```python
from build123d import *

# Parameters (mm, degrees)
F0_R            = 150
F1_DEPTH        = 15
F3_DEPTH        = 15.001
F3_COPIES_COUNT = 6
F5_DEPTH        = 3
F5_COPIES_COUNT = 6
F6_R            = 25
F6_R_2          = 11.35
F7_DEPTH        = 3
F8_DEPTH        = 15.001


# Not quite as in the source:
# - an extrude ends at something that could not be found from the text; its depth is read off the source's solid
# - a pattern or mirror of a feature is missing from the dataset's text; its kind, count and spacing are read off the source's solid


with BuildPart() as f1:
    # F0 (on Top) → F1 (new body)
    with BuildSketch(Plane.XY):
        Circle(F0_R)
    extrude(amount=F1_DEPTH)

    # F2 (on face) → F3 (cut, through all)
    with BuildSketch(Plane.XY.offset(15)):
        with BuildLine():
            ThreePointArc((0, 120), (-5.3033008589, 117.8033008589), (-7.5, 112.5))
            Line((-7.5, 112.5), (-7.5, 27.5))
            ThreePointArc((-7.5, 27.5), (-5.3033008589, 22.1966991411), (0, 20))
            Line((0, 20), (0, 120))
        make_face()
        with BuildLine():
            ThreePointArc((7.5, 112.5), (5.3033008589, 117.8033008589), (0, 120))
            Line((0, 120), (0, 20))
            ThreePointArc((0, 20), (5.3033008589, 22.1966991411), (7.5, 27.5))
            Line((7.5, 27.5), (7.5, 112.5))
        make_face()
    f3 = extrude(amount=-F3_DEPTH, mode=Mode.SUBTRACT)

    # F3_copies: F3 ×6 about axis
    f3_copies_axis = Axis((0, 0, 0), (0, 0, 1))
    for i in range(1, F3_COPIES_COUNT):
        add(f3.rotate(f3_copies_axis, i * 360 / F3_COPIES_COUNT), mode=Mode.SUBTRACT)

    # F4 (on face) → F5 (cut)
    with BuildSketch(Plane.XY.offset(15)):
        with BuildLine():
            Line((13.85, 27.5), (13.85, 112.5))
            ThreePointArc((13.85, 112.5), (0, 126.35), (-13.85, 112.5))
            Line((-13.85, 112.5), (-13.85, 27.5))
            ThreePointArc((-13.85, 27.5), (0, 13.65), (13.85, 27.5))
        make_face()
        with BuildLine():
            Line((7.5, 112.5), (7.5, 27.5))
            ThreePointArc((7.5, 27.5), (0, 20), (-7.5, 27.5))
            Line((-7.5, 27.5), (-7.5, 112.5))
            ThreePointArc((-7.5, 112.5), (0, 120), (7.5, 112.5))
        make_face(mode=Mode.SUBTRACT)
    f5 = extrude(amount=-F5_DEPTH, mode=Mode.SUBTRACT)

    # F5_copies: F5 ×6 about axis
    f5_copies_axis = Axis((0, 0, 0), (0, 0, 1))
    for i in range(1, F5_COPIES_COUNT):
        add(f5.rotate(f5_copies_axis, i * 360 / F5_COPIES_COUNT), mode=Mode.SUBTRACT)

    # F6 (on face) → F7 (cut, through all)
    with BuildSketch(Plane.XY.offset(15)):
        Circle(F6_R)
        with BuildLine():
            ThreePointArc((11.0771869157, 19.186250543), (11.8212467617, 6.825), (22.1543738315, 0))
            ThreePointArc((22.1543738315, 0), (11.8212467617, -6.825), (11.0771869157, -19.186250543))
            ThreePointArc((11.0771869157, -19.186250543), (0, -13.65), (-11.0771869157, -19.186250543))
            ThreePointArc((-11.0771869157, -19.186250543), (-11.8212467617, -6.825), (-22.1543738315, 0))
            ThreePointArc((-22.1543738315, 0), (-11.8212467617, 6.825), (-11.0771869157, 19.186250543))
            ThreePointArc((-11.0771869157, 19.186250543), (0, 13.65), (11.0771869157, 19.186250543))
        make_face(mode=Mode.SUBTRACT)
        with BuildLine():
            ThreePointArc((11.0771869157, -19.186250543), (11.8212467617, -6.825), (22.1543738315, 0))
            ThreePointArc((22.1543738315, 0), (11.8212467617, 6.825), (11.0771869157, 19.186250543))
            ThreePointArc((11.0771869157, 19.186250543), (0, 13.65), (-11.0771869157, 19.186250543))
            ThreePointArc((-11.0771869157, 19.186250543), (-11.8212467617, 6.825), (-22.1543738315, 0))
            ThreePointArc((-22.1543738315, 0), (-11.8212467617, -6.825), (-11.0771869157, -19.186250543))
            ThreePointArc((-11.0771869157, -19.186250543), (0, -13.65), (11.0771869157, -19.186250543))
        make_face()
        Circle(F6_R_2, mode=Mode.SUBTRACT)
        Circle(F6_R_2)
    extrude(amount=-F7_DEPTH, mode=Mode.SUBTRACT)

    # F6 (on face) → F8 (cut, through all)
    with BuildSketch(Plane.XY.offset(15)):
        Circle(F6_R_2)
    extrude(amount=-F8_DEPTH, mode=Mode.SUBTRACT)


solid = f1.part
```
CAD build for the part. Positions are in the model's coordinates, mm. A direction names the side the tool comes from. Coordinates: 2 decimals unless noted, no trailing zeros. Order: outer loops, then holes, each group sorted by start corner. A loop starts at its lowest first (then second) coordinate and runs counter-clockwise, first axis right, second up. Notation, with made-up numbers: (42.25, 21) -> (49.25, 21) arc R22 ccw to (49.25, 54) -> close; hole circle Ø9 at (-4, 55.25). An arc over 180 degrees is marked (long way). Use one line per item in the form item = value. Start each with the question number.
1) Pull direction X, two halves, no side cores. Call faces 4 (the cylindrical face through (10.485, -4.347, 6.084)), 5 (the cylindrical face through (-19.527, 148.724, 7.395)), 6 (the flat face through (31, 2, 0)): +X half, -X half, draft (parallel to the pull), parting line (faces both ways), or undercut.
2) Band-saw the part on D-D on x = 57.5. Give the cut face in (y, z), then the cut area to 3 significant figures.
3) Band-saw the part on C-C on z = 5.5. Give the cut face in (x, y), then the cut area to 3 significant figures.
4) Drill centre lines: L1, parallel to Y at x = 0, z = 9.75; L2, parallel to Y at x = -59, z = 8.5; L3, parallel to Y at x = 81, z = 9. Where is each one in solid material? Low to high. Write a range as [from, to].
5) Band-saw the part on A-A on x = 0. Give the cut face in (y, z), then the cut area to 3 significant figures.
6) Drop flat-ended pins along their axis: pin 1 (3.5 mm diameter, centred on y = -55.5, z = 13, fed in from -X); pin 2 (4 mm diameter, centred on x = 106, z = 7, fed in from +Y); pin 3 (3.5 mm diameter, centred on y = 90.5, z = 13.5, fed in from -X); pin 4 (2 mm diameter, centred on x = -100.5, y = -68, fed in from -Z). Give the stop position or say it passes through.
7) Band-saw the part on B-B on y = -81. Give the cut face in (x, z).
8) Tool access for faces 1 (the flat face through (68.06, -23.3, 13.52)), 2 (the flat face through (-35, 2, 15)), 3 (the flat face through (7.5, 69, 6)): list every direction of +Z, -Z, +X, -X, +Y, -Y with a clear straight run to the whole face (end or side of a thin tool).
Entries:
q1.face_4 = undercut
q1.face_5 = parting line
q1.face_6 = draft
q2.outline = (-138.54, 0) -> (-41.86, 0) -> (-41.86, 12) -> (-49.19, 12) -> (-49.19, 15) -> (-138.54, 15) -> close; (-24.54, 0) -> (24.54, 0) -> (24.54, 12) -> (17.21, 12) -> (17.21, 15) -> (-17.21, 15) -> (-17.21, 12) -> (-24.54, 12) -> close; (41.86, 0) -> (138.54, 0) -> (138.54, 15) -> (49.19, 15) -> (49.19, 12) -> (41.86, 12) -> close
q2.area = 3,550 mm2
q3.outline = circle Ø300 at (0, 0); hole (-101.18, -49.75) arc R7.5 ccw to (-93.68, -62.75) -> (-20.07, -20.25) arc R7.5 ccw to (-27.57, -7.25) -> close; hole (-101.18, 49.75) -> (-27.57, 7.25) arc R7.5 ccw to (-20.07, 20.25) -> (-93.68, 62.75) arc R7.5 ccw to start; hole circle Ø22.7 at (0, 0); hole (-7.5, -112.5) arc R7.5 ccw to (7.5, -112.5) -> (7.5, -27.5) arc R7.5 ccw to (-7.5, -27.5) -> close; hole (-7.5, 27.5) arc R7.5 ccw to (7.5, 27.5) -> (7.5, 112.5) arc R7.5 ccw to (-7.5, 112.5) -> close; hole (20.07, -20.25) -> (93.68, -62.75) arc R7.5 ccw to (101.18, -49.75) -> (27.57, -7.25) arc R7.5 ccw to start; hole (20.07, 20.25) arc R7.5 ccw to (27.57, 7.25) -> (101.18, 49.75) arc R7.5 ccw to (93.68, 62.75) -> close
q3.area = 61,600 mm2
q4.L1 = [-150, -120], [-20, -11.35], [11.35, 20], [120, 150]
q4.L2 = [-137.91, -42.72], [-25.4, 25.4], [42.72, 137.91]
q4.L3 = [-126.25, -55.43], [-38.11, 38.11], [55.43, 126.25]
q5.outline = (-150, 0) -> (-120, 0) -> (-120, 12) -> (-126.35, 12) -> (-126.35, 15) -> (-150, 15) -> close; (-20, 0) -> (-11.35, 0) -> (-11.35, 12) -> (-20, 12) -> close; (11.35, 0) -> (20, 0) -> (20, 12) -> (11.35, 12) -> close; (120, 0) -> (150, 0) -> (150, 15) -> (126.35, 15) -> (126.35, 12) -> (120, 12) -> close
q5.area = 1,070 mm2
q6.pin_1 = -140.04
q6.pin_2 = 108.09
q6.pin_3 = -120.93
q6.pin_4 = 0
q7.outline = (-126.25, 0) -> (-7.5, 0) -> (-7.5, 12) -> (-13.85, 12) -> (-13.85, 15) -> (-126.25, 15) -> close; (7.5, 0) -> (126.25, 0) -> (126.25, 15) -> (13.85, 15) -> (13.85, 12) -> (7.5, 12) -> close
q8.face_1 = +Z
q8.face_2 = +Z, +X, -X, +Y, -Y
q8.face_3 = +Z, -Z
